Can you work these out from the drawing? Everything is in mm from the part's minimum corner. Give positions to 0.01 mm unless a question says otherwise; leave off trailing zeros. Write each loop counter-clockwise with the first axis right and the second up, starting at its lowest first coordinate (ties: lowest second). Pieces come first, ordered by that corner, then holes. Notation, with made-up numbers: (-8.75, -39.5) - (44.25, -39.5) arc R15 cw to (44.25, -17.5) - close; hole circle Ø9 at (-22, 13.5). An arc over 180 degrees is marked (long way). Use a Markdown table: item, result.
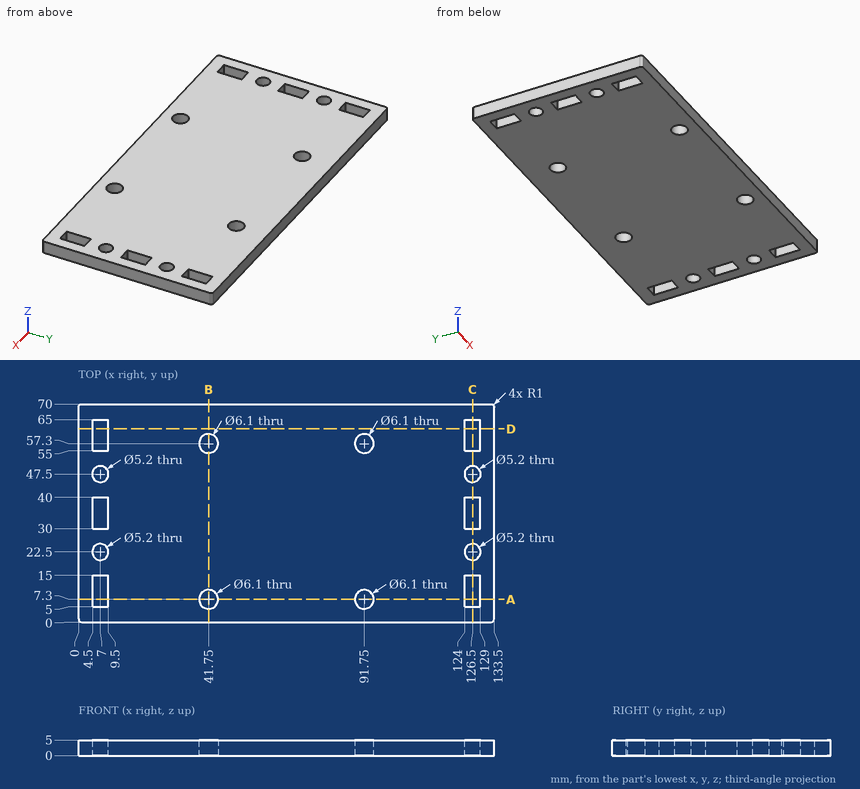
Item 1: If we section it at A-A, the plane y = 7.3: Write out the boundary of the cut face in (x, z).
Values:
| item | result |
|---|---|
| outline | (0, 0) - (4.5, 0) - (4.5, 5) - (0, 5) - close; (9.5, 0) - (38.7, 0) - (38.7, 5) - (9.5, 5) - close; (44.8, 0) - (88.7, 0) - (88.7, 5) - (44.8, 5) - close; (94.8, 0) - (124, 0) - (124, 5) - (94.8, 5) - close; (129, 0) - (133.5, 0) - (133.5, 5) - (129, 5) - close |
Item 2: If we section it at D-D, the plane y = 62: Write out the boundary of the cut face in (x, z).
Values:
| item | result |
|---|---|
| outline | (0, 0) - (4.5, 0) - (4.5, 5) - (0, 5) - close; (9.5, 0) - (124, 0) - (124, 5) - (9.5, 5) - close; (129, 0) - (133.5, 0) - (133.5, 5) - (129, 5) - close |
Item 3: If we section it at B-B, the plane x = 41.75: Write out the boundary of the cut face in (y, z), plus the area to 3 significant figures.
Values:
| item | result |
|---|---|
| outline | (0, 0) - (4.25, 0) - (4.25, 5) - (0, 5) - close; (10.35, 0) - (54.25, 0) - (54.25, 5) - (10.35, 5) - close; (60.35, 0) - (70, 0) - (70, 5) - (60.35, 5) - close |
| area | 289 mm2 |
Item 4: I need wall thicknesses on line 1 along X through (y, z) = (62, 2.2); line 2 along Y through (x, z) = (41.75, 3.7); line 3 along Y through (x, z) = (7, 3.7). Which ranges of each line are inside material? Lowest first, please. Write a range as [from, to].
Values:
| item | result |
|---|---|
| line 1 | x = [0, 4.5], [9.5, 124], [129, 133.5] |
| line 2 | y = [0, 4.25], [10.35, 54.25], [60.35, 70] |
| line 3 | y = [0, 5], [15, 19.9], [25.1, 30], [40, 44.9], [50.1, 55], [65, 70] |
Item 5: If we section it at C-C, the plane x = 126.5: Write out the boundary of the cut face in (y, z).
Values:
| item | result |
|---|---|
| outline | (0, 0) - (5, 0) - (5, 5) - (0, 5) - close; (15, 0) - (19.9, 0) - (19.9, 5) - (15, 5) - close; (25.1, 0) - (30, 0) - (30, 5) - (25.1, 5) - close; (40, 0) - (44.9, 0) - (44.9, 5) - (40, 5) - close; (50.1, 0) - (55, 0) - (55, 5) - (50.1, 5) - close; (65, 0) - (70, 0) - (70, 5) - (65, 5) - close |
